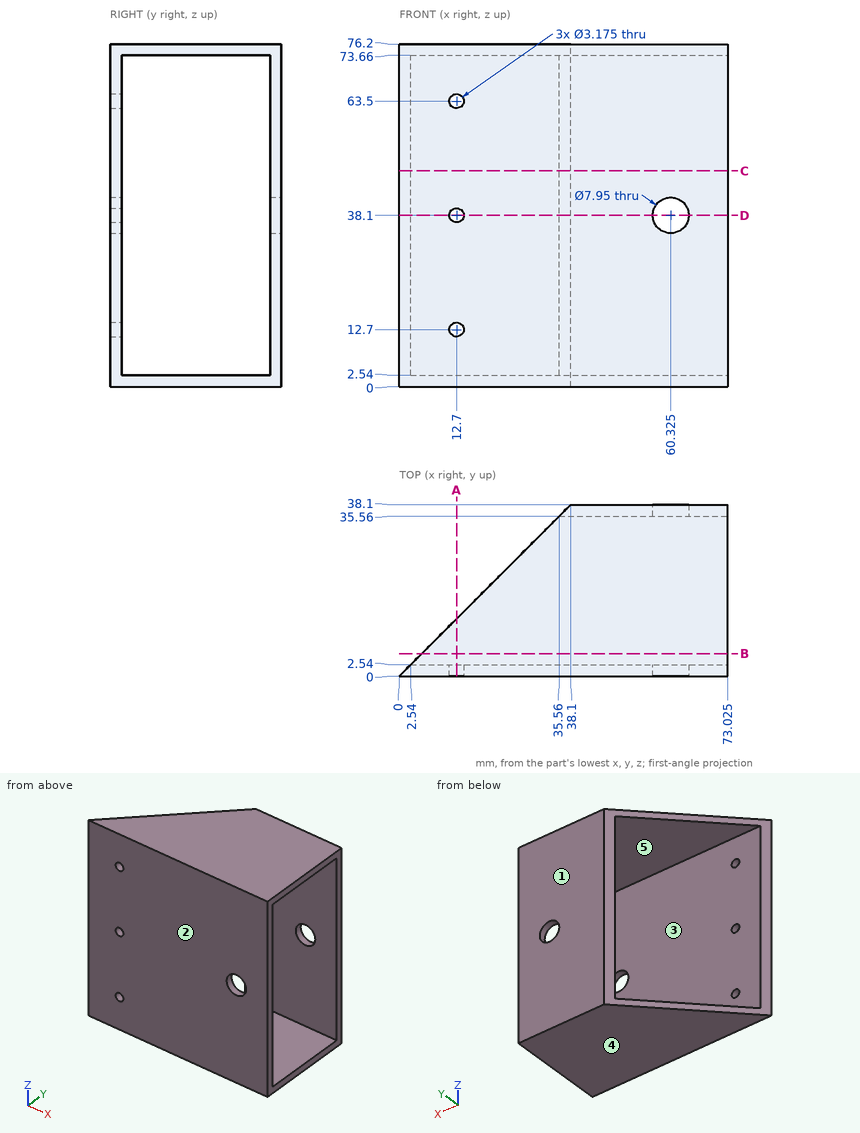
The figure shows three views and two pictorial views of one solid part (mm, origin at its lowest corner). Answer the questions. A direction names the side the tool comes from. Round coordinates to 2 decimals unless told otherwise and drop trailing zeros. Order: outer loops, then holes, each group sorted by start corner. A loop starts at its lowest first (then second) coordinate and runs counter-clockwise, first axis right, second up. Notation, with made-up numbers: M 66,-14 L 118,-14 A8 cw 118,-3 Z; hole C 32.25,79 d7. An arc over 180 degrees is marked long. Put each result on its own line as item: value. Start each with the question number.
Q1. Section D-D, the plane z = 38.1 is taken. Give the number of separate pieces and of enclosed holes in the cut face, and give its area (3 significant figures).
Q2. For a pull along Y with two mould halves and no side action, classify the marked faces 1, 2 and 3 as pulls with the +Y half, pulls with the -Y half, needs draft (parallel to the pull), parting line crosses it, or undercut.
Q3. Flat-ended cylindrical pins translate along their axes: pin 1 (18.5 mm diameter, centred on x = 47, z = 33, fed in from -Y); pin 2 (7 mm diameter, centred on x = 60.325, z = 38.1, fed in from -Y); pin 3 (4 mm diameter, centred on x = 12, z = 16.5, fed in from +Y). Find the tip coordinate at first contact, or state that the pin passes through.
Q4. Section B-B, the plane y = 5 is taken. Write down the section's boundary in (x, z) (3 decimals).
Q5. A tool of negligible diameter and unlimited length cuts with its end or side. For the marked faces 4 and 5, from which of +Z, -Z, +X, -X, +Y, -Y can it reach the whole face along a straight path? Write none if from no direction.
Q6. Section C-C, the plane z = 48 is taken. Write down the section's boundary in (x, y) (3 decimals).
Q7. Straight lines are drawn through the part: L1, parallel to Z at x = 32, y = 11; L2, parallel to Y at x = 39.5, z = 68; L3, parallel to Z at x = 12.7, y = 1.05. For each, find the intervals that lie inside material, in ascending order. Write a range as [from, to].
Q8. Section A-A, the plane x = 12.7 is taken. Write down the section's boundary in (y, z), and give its area (3 significant figures).
Findings below:
1. separate pieces: 5
1. enclosed holes: 0
1. area: 226 mm^2
2. face 1: pulls with the +Y half
2. face 2: pulls with the -Y half
2. face 3: undercut
3. pin 1: stops at y = 0
3. pin 2: passes through
3. pin 3: stops at y = 2.54
4. outline: M 5,0 L 73.025,0 L 73.025,2.54 L 5,2.54 Z; M 5,73.66 L 73.025,73.66 L 73.025,76.2 L 5,76.2 Z
5. face 4: -Z, +X, -X, +Y, -Y
5. face 5: +X, -X
6. outline: M 0,0 L 73.025,0 L 73.025,2.54 L 2.54,2.54 Z; M 35.56,35.56 L 73.025,35.56 L 73.025,38.1 L 38.1,38.1 Z
7. L1: z = [0, 2.54], [73.66, 76.2]
7. L2: y = [0, 2.54], [35.56, 38.1]
7. L3: z = [0, 11.11], [14.29, 36.51], [39.69, 61.91], [65.09, 76.2]
8. outline: M 0,0 L 12.7,0 L 12.7,2.54 L 2.54,2.54 L 2.54,11.11 L 0,11.11 Z; M 0,14.29 L 2.54,14.29 L 2.54,36.51 L 0,36.51 Z; M 0,39.69 L 2.54,39.69 L 2.54,61.91 L 0,61.91 Z; M 0,65.09 L 2.54,65.09 L 2.54,73.66 L 12.7,73.66 L 12.7,76.2 L 0,76.2 Z
8. area: 221 mm^2
